Part model, mm, in its own coordinate system. Face numbers are marked on the shaded views. A direction names the side the tool comes from. Coordinates: 2 decimals unless noted, no trailing zeros. Write each loop counter-clockwise with the first axis right and the second up, starting at its lowest first coordinate (ties: lowest second). Pieces come first, ordered by that corner, then holes. Notation, with made-up numbers: (-6.5, 24) -> (-2.5, 24) arc R25 cw to (-2.5, 37) -> close; hole circle Ø5 at (67, 49). An arc over 180 degrees is marked (long way). Write item = value, one per line.
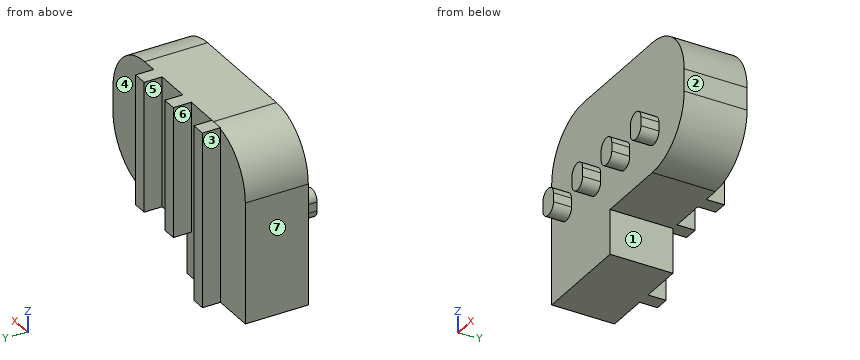
from build123d import *

# Parameters (mm, degrees)
SKETCH_1_W      = 12.5
SKETCH_1_H      = 7.25
EXTRUDE_1_DEPTH = 3.5
FILLET_1_R      = 3
SKETCH_2_W      = 5.5
SKETCH_2_H      = 2.5
EXTRUDE_2_DEPTH = 3.5
SKETCH_3_W      = 0.8
SKETCH_3_H      = 9.746247653
SKETCH_3_H_2    = 7.25
EXTRUDE_3_DEPTH = 1
EXTRUDE_4_DEPTH = 1


with BuildPart() as part:
    # 草图1 → 凸台-拉伸1 (new body)
    with BuildSketch(Plane(origin=(0, 0, 0), x_dir=(1, 0, 0), z_dir=(0, 1, 0))):
        with Locations((6.25, 3.625)):
            Rectangle(SKETCH_1_W, SKETCH_1_H)
    extrude(amount=EXTRUDE_1_DEPTH)

    # 圆角1
    fillet_1_edges = [part.edges().sort_by_distance(p)[0] for p in [
        (12.5, 1.75, -7.25),
        (12.5, 1.75, 0),
        (0, 1.75, 0),
    ]]
    fillet(fillet_1_edges, radius=FILLET_1_R)

    # 草图2 → 凸台-拉伸2 (add)
    with BuildSketch(Plane(origin=(0, 3.5, 0), x_dir=(1, 0, 0), z_dir=(0, 1, 0))):
        with Locations((2.75, 8.5)):
            Rectangle(SKETCH_2_W, SKETCH_2_H)
    extrude(amount=-EXTRUDE_2_DEPTH)

    # 草图3 → 凸台-拉伸3 (add)
    with BuildSketch(Plane(origin=(0, 3.5, 0), x_dir=(1, 0, 0), z_dir=(0, 1, 0))):
        with Locations((2.75, 4.876876174)):
            Rectangle(SKETCH_3_W, SKETCH_3_H)
        with Locations((5.5, 3.625)):
            Rectangle(SKETCH_3_W, SKETCH_3_H_2)
        with Locations((8.25, 3.625)):
            Rectangle(SKETCH_3_W, SKETCH_3_H_2)
    extrude(amount=EXTRUDE_3_DEPTH)

    # 草图6 → 凸台-拉伸4 (add)
    with BuildSketch(Plane.XZ):
        with BuildLine():
            Line((6.365, -4.75), (6.365, -5.25))
            ThreePointArc((6.365, -5.25), (6.865, -5.75), (7.365, -5.25))
            Line((7.365, -5.25), (7.365, -4.75))
            ThreePointArc((7.365, -4.75), (6.865, -4.25), (6.365, -4.75))
        make_face()
        with BuildLine():
            Line((9.115, -4.75), (9.115, -5.25))
            ThreePointArc((9.115, -5.25), (9.615, -5.75), (10.115, -5.25))
            Line((10.115, -5.25), (10.115, -4.75))
            ThreePointArc((10.115, -4.75), (9.615, -4.25), (9.115, -4.75))
        make_face()
        with BuildLine():
            Line((4.615, -5.25), (4.615, -4.75))
            ThreePointArc((4.615, -4.75), (4.115, -4.25), (3.615, -4.75))
            Line((3.615, -4.75), (3.615, -5.25))
            ThreePointArc((3.615, -5.25), (4.115, -5.75), (4.615, -5.25))
        make_face()
        with BuildLine():
            Line((0.865, -4.75), (0.865, -5.25))
            ThreePointArc((0.865, -5.25), (1.365, -5.75), (1.865, -5.25))
            Line((1.865, -5.25), (1.865, -4.75))
            ThreePointArc((1.865, -4.75), (1.365, -4.25), (0.865, -4.75))
        make_face()
    extrude(amount=EXTRUDE_4_DEPTH)


solid = part.part
Q1. Pin check, flat tips, straight feed: pin 1 (0.5 mm diameter, centred on y = 4, z = -5.5, fed in from +X); pin 2 (1 mm diameter, centred on x = 3.5, z = -2.5, fed in from -Y); pin 3 (3 mm diameter, centred on y = 2.5, z = -8.5, fed in from +X). Stop position of each tip, or through.
Model answer:
pin_1 = 8.65
pin_2 = 0
pin_3 = 10.7
Q2. Which spindle directions (+Z, -Z, +X, -X, +Y, -Y) get a long thin tool onto all of the face, cutting with end or side? Do the marked faces 1, 2 and 3. Say none if no direction does.
Model answer:
face_1 = -Z, +X, +Y, -Y
face_2 = +Z, -Z, +X, +Y, -Y
face_3 = +Z, -Z, -X, +Y
Q3. Mould opens along X. For the marked faces 4, 5, 6 and 7 say: released by +X, released by -X, zero draft, split by the parting line, or undercut.
Model answer:
face_4 = zero draft
face_5 = undercut
face_6 = undercut
face_7 = released by -X
Q4. Saw through at D-D on y = 3. Give the cut face in (x, z), and give its area (3 significant figures).
Model answer:
outline = (0, -9.75) -> (5.5, -9.75) -> (5.5, -7.25) -> (9.5, -7.25) arc R3 ccw to (12.5, -4.25) -> (12.5, -3) arc R3 ccw to (9.5, 0) -> (3, 0) arc R3 ccw to (0, -3) -> close
area = 98.6 mm²
Q5. Saw through at C-C on y = -0.55. Give the cut face in (x, z) (3 decimals), and give its area (3 significant figures).
Model answer:
outline = (0.865, -5.25) arc R0.5 ccw to (1.865, -5.25) -> (1.865, -4.75) arc R0.5 ccw to (0.865, -4.75) -> close; (3.615, -5.25) arc R0.5 ccw to (4.615, -5.25) -> (4.615, -4.75) arc R0.5 ccw to (3.615, -4.75) -> close; (6.365, -5.25) arc R0.5 ccw to (7.365, -5.25) -> (7.365, -4.75) arc R0.5 ccw to (6.365, -4.75) -> close; (9.115, -5.25) arc R0.5 ccw to (10.115, -5.25) -> (10.115, -4.75) arc R0.5 ccw to (9.115, -4.75) -> close
area = 5.14 mm²
Q6. Probe line 1 (X direction, y = 4.1, z = -4.75); line 2 (Y direction, x = 10.75, z = -3); line 3 (X direction, y = 0.4, z = -8.75). List the from-to ranges inside material, lowest first. Write a range as from..to.
Model answer:
line_1 = 2.35..3.15, 5.1..5.9, 7.85..8.65
line_2 = 0..3.5
line_3 = 0..5.5
Q7. Saw through at A-A on y = 4.1. Give the cut face in (x, z), and give its area (3 significant figures).
Model answer:
outline = (2.35, -9.75) -> (3.15, -9.75) -> (3.15, 0) -> (2.35, 0) -> close; (5.1, -7.25) -> (5.9, -7.25) -> (5.9, 0) -> (5.1, 0) -> close; (7.85, -7.25) -> (8.65, -7.25) -> (8.65, 0) -> (7.85, 0) -> close
area = 19.4 mm²
Q8. Saw through at B-B on z = -4. Give the cut face in (x, y).
Model answer:
outline = (0, 0) -> (12.5, 0) -> (12.5, 3.5) -> (8.65, 3.5) -> (8.65, 4.5) -> (7.85, 4.5) -> (7.85, 3.5) -> (5.9, 3.5) -> (5.9, 4.5) -> (5.1, 4.5) -> (5.1, 3.5) -> (3.15, 3.5) -> (3.15, 4.5) -> (2.35, 4.5) -> (2.35, 3.5) -> (0, 3.5) -> close
